```python
from build123d import *

# Parameters (mm, degrees)
EXTRUDE_1_DEPTH        = 8
SKETCH_2_W             = 101.5
SKETCH_2_H             = 90.5
PCB_DEPTH              = 1.62
CUT_EXTRUDE_1931_REACH = 77.575
SKETCH_2_4_W           = 102
SKETCH_2_4_H           = 61
SKETCH_2_5_W           = 107
SKETCH_2_5_H           = 68.5
CUT_EXTRUDE_1995_DEPTH = 5.85
SKETCH_3_W             = 101.5
SKETCH_3_H             = 14
CUT_EXTRUDE_2361_DEPTH = 2.5
SKETCH_3_3_W           = 46
SKETCH_3_3_H           = 2
CUT_EXTRUDE_2_DEPTH    = 2.5
SKETCH_2585_R          = 2.15
CUT_EXTRUDE_2883_DEPTH = 2.2
SKETCH_3_2_R           = 1.15
CUT_EXTRUDE_2937_DEPTH = 76.574880086
FILLET_1_R             = 3
SKETCH_2_6_R           = 0.625
LED_DEPTH              = 76.574880086
PCB_START              = -1.62
SKETCH_2_7_W           = 54
SKETCH_2_7_H           = 4
PCB_2_DEPTH            = 1.62


with BuildPart() as part:
    # 草图1 → 凸台-拉伸1 (new body)
    with BuildSketch(Plane(origin=(0, 0, 0), x_dir=(1, 0, 0), z_dir=(0, 1, 0))):
        Polygon((57, 45.25), (60, 45.25), (60, 42.25), (60, -42.25), (60, -45.25), (57, -45.25), (-57, -45.25), (-60, -45.25), (-60, -42.25), (-60, 42.25), (-60, 45.25), (-57, 45.25), align=None)
    extrude(amount=EXTRUDE_1_DEPTH)

    # 草图2 → PCB (cut)
    with BuildSketch(Plane(origin=(0, 8, 0), x_dir=(1, 0, 0), z_dir=(0, 1, 0))):
        with Locations((2.75, 0)):
            Rectangle(SKETCH_2_W, SKETCH_2_H)
    extrude(amount=-PCB_DEPTH, mode=Mode.SUBTRACT)

    # 草图2<4> → Cut-Extrude 1931 (cut, up to next)
    with BuildSketch(Plane(origin=(0, 8, 0), x_dir=(1, 0, 0), z_dir=(0, 1, 0)), mode=Mode.PRIVATE) as cut_extrude_1931_sk1:
        with Locations((0, -5.25)):
            Rectangle(SKETCH_2_4_W, SKETCH_2_4_H)
    cut_extrude_1931_tool1 = extrude(cut_extrude_1931_sk1.sketch, amount=-CUT_EXTRUDE_1931_REACH, mode=Mode.PRIVATE) & part.part
    add(cut_extrude_1931_tool1.solids().sort_by_distance((0, 8, 5.25))[0], mode=Mode.SUBTRACT)

    # 草图2<5> → Cut-Extrude 1995 (cut)
    with BuildSketch(Plane(origin=(0, 8, 0), x_dir=(1, 0, 0), z_dir=(0, 1, 0))):
        with Locations((0, -7)):
            Rectangle(SKETCH_2_5_W, SKETCH_2_5_H)
    extrude(amount=-CUT_EXTRUDE_1995_DEPTH, mode=Mode.SUBTRACT)

    # Sketch 3 → Cut-Extrude 2361 (cut)
    with BuildSketch(Plane(origin=(0, 6.38, 0), x_dir=(1, 0, 0), z_dir=(0, 1, 0))):
        with Locations((2.75, 34.25)):
            Rectangle(SKETCH_3_W, SKETCH_3_H)
    extrude(amount=-CUT_EXTRUDE_2361_DEPTH, mode=Mode.SUBTRACT)

    # 草图3<3> → 穿孔焊盘切除2 (cut)
    with BuildSketch(Plane(origin=(0, 6.38, 0), x_dir=(1, 0, 0), z_dir=(0, 1, 0))):
        with Locations((-17, 42.25)):
            Rectangle(SKETCH_3_3_W, SKETCH_3_3_H)
    extrude(amount=-CUT_EXTRUDE_2_DEPTH, mode=Mode.SUBTRACT)

    # Sketch 2585 → Cut-Extrude 2883 (cut)
    with BuildSketch(Plane(origin=(0, 0, 0), x_dir=(1, 0, 0), z_dir=(0, 1, 0))):
        with Locations(Location((-56.5, -41.75, 0), (0, 0, 270))):
            Circle(SKETCH_2585_R)
        with Locations(Location((-56.5, 41.75, 0), (0, 0, 270))):
            Circle(SKETCH_2585_R)
        with Locations(Location((56.5, 41.75, 0), (0, 0, 270))):
            Circle(SKETCH_2585_R)
        with Locations(Location((56.5, -41.75, 0), (0, 0, 270))):
            Circle(SKETCH_2585_R)
    extrude(amount=CUT_EXTRUDE_2883_DEPTH, mode=Mode.SUBTRACT)

    # Sketch 3 2 → Cut-Extrude 2937 (cut, through all)
    with BuildSketch(Plane(origin=(0, 0, 0), x_dir=(1, 0, 0), z_dir=(0, 1, 0))):
        with Locations(Location((-56.5, -41.75, 0), (0, 0, 270))):
            Circle(SKETCH_3_2_R)
        with Locations(Location((-56.5, 41.75, 0), (0, 0, 270))):
            Circle(SKETCH_3_2_R)
        with Locations(Location((56.5, 41.75, 0), (0, 0, 270))):
            Circle(SKETCH_3_2_R)
        with Locations(Location((56.5, -41.75, 0), (0, 0, 270))):
            Circle(SKETCH_3_2_R)
    extrude(amount=CUT_EXTRUDE_2937_DEPTH, mode=Mode.SUBTRACT)

    # 圆角1
    # the kernel refuses this fillet: 3 mm, written as the material it adds along each edge
    with BuildSketch(Plane(origin=(-51, 2.15, -25.25), x_dir=(1, 0, 0), z_dir=(0, -1, 0)), Plane(origin=(-51, 2.15, 35.75), x_dir=(0, 0, -1), z_dir=(0, -1, 0))) as fillet_1_piece_1:
        with BuildLine():
            CenterArc((FILLET_1_R, FILLET_1_R), FILLET_1_R, 180, 90)
            Line((0, FILLET_1_R), (0, 0))
            Line((0, 0), (FILLET_1_R, 0))
        make_face()
    extrude(amount=2.15)
    with BuildSketch(Plane(origin=(-53.5, 8, -27.25), x_dir=(1, 0, 0), z_dir=(0, -1, 0))) as fillet_1_piece_2:
        with BuildLine():
            CenterArc((FILLET_1_R, FILLET_1_R), FILLET_1_R, 180, 90)
            Line((0, FILLET_1_R), (0, 0))
            Line((0, 0), (FILLET_1_R, 0))
        make_face()
    extrude(amount=5.85)
    with BuildSketch(Plane(origin=(-53.5, 8, 41.25), x_dir=(1, 0, 0), z_dir=(0, -1, 0))) as fillet_1_piece_3:
        with BuildLine():
            CenterArc((FILLET_1_R, -FILLET_1_R), FILLET_1_R, 90, 90)
            Line((0, -FILLET_1_R), (0, 0))
            Line((0, 0), (FILLET_1_R, 0))
        make_face()
    extrude(amount=5.85)
    with BuildSketch(Plane(origin=(51, 2.15, 35.75), x_dir=(0, 0, -1), z_dir=(0, -1, 0)), Plane(origin=(51, 2.15, -25.25), x_dir=(-1, 0, 0), z_dir=(0, -1, 0))) as fillet_1_piece_4:
        with BuildLine():
            CenterArc((FILLET_1_R, -FILLET_1_R), FILLET_1_R, 90, 90)
            Line((0, -FILLET_1_R), (0, 0))
            Line((0, 0), (FILLET_1_R, 0))
        make_face()
    extrude(amount=2.15)
    with BuildSketch(Plane(origin=(53.5, 6.38, 41.25), x_dir=(0, 0, -1), z_dir=(0, -1, 0))) as fillet_1_piece_5:
        with BuildLine():
            CenterArc((FILLET_1_R, -FILLET_1_R), FILLET_1_R, 90, 90)
            Line((0, -FILLET_1_R), (0, 0))
            Line((0, 0), (FILLET_1_R, 0))
        make_face()
    extrude(amount=4.23)
    with BuildSketch(Plane(origin=(53.5, 3.88, -27.25), x_dir=(0, 0, 1), z_dir=(0, -1, 0))) as fillet_1_piece_6:
        with BuildLine():
            CenterArc((FILLET_1_R, FILLET_1_R), FILLET_1_R, 180, 90)
            Line((0, FILLET_1_R), (0, 0))
            Line((0, 0), (FILLET_1_R, 0))
        make_face()
    extrude(amount=1.73)
    with BuildSketch(Plane(origin=(6, 6.38, -43.25), x_dir=(-1, 0, 0), z_dir=(0, -1, 0))) as fillet_1_piece_7:
        with BuildLine():
            CenterArc((2.828427125, -3), FILLET_1_R, 90, 70.528779366)
            Line((0, -2), (0, 0))
            Line((0, 0), (2.828427125, 0))
        make_face()
    extrude(amount=2.5)
    with BuildSketch(Plane(origin=(-40, 6.38, -43.25), x_dir=(0, 0, 1), z_dir=(0, -1, 0))) as fillet_1_piece_8:
        with BuildLine():
            CenterArc((3, -2.828427125), FILLET_1_R, 109.471220634, 70.528779366)
            Line((0, -2.828427125), (0, 0))
            Line((0, 0), (2, 0))
        make_face()
    extrude(amount=2.5)
    with BuildSketch(Plane(origin=(-48, 6.38, -41.25), x_dir=(0, 0, 1), z_dir=(0, -1, 0))) as fillet_1_piece_9:
        with BuildLine():
            CenterArc((FILLET_1_R, -FILLET_1_R), FILLET_1_R, 90, 90)
            Line((0, -FILLET_1_R), (0, 0))
            Line((0, 0), (FILLET_1_R, 0))
        make_face()
    extrude(amount=2.5)
    with BuildSketch(Plane(origin=(53.5, 6.38, -41.25), x_dir=(0, 0, 1), z_dir=(0, -1, 0))) as fillet_1_piece_10:
        with BuildLine():
            CenterArc((FILLET_1_R, FILLET_1_R), FILLET_1_R, 180, 90)
            Line((0, FILLET_1_R), (0, 0))
            Line((0, 0), (FILLET_1_R, 0))
        make_face()
    extrude(amount=2.5)

    # 草图2<6> → LED孔 (cut, through all)
    with BuildSketch(Plane(origin=(0, 8, 0), x_dir=(1, 0, 0), z_dir=(0, 1, 0))):
        with Locations(Location((0.295, 40.636, 0), (0, 0, 270))):
            Circle(SKETCH_2_6_R)
        with Locations(Location((-27.9, 40.636, 0), (0, 0, 270))):
            Circle(SKETCH_2_6_R)
    extrude(amount=-LED_DEPTH, mode=Mode.SUBTRACT)

    # 草图2<7> → PCB 2 (add)
    with BuildSketch(Plane(origin=(0, 8, 0), x_dir=(1, 0, 0), z_dir=(0, 1, 0)).offset(PCB_START)):
        with Locations((8.5, -43.25)):
            Rectangle(SKETCH_2_7_W, SKETCH_2_7_H)
    extrude(amount=PCB_2_DEPTH)


solid = part.part
```
Work out the finished part from the listing and answer in its coordinate system (mm). A direction names the side the tool comes from. Round coordinates to 2 decimals unless told otherwise and drop trailing zeros. Loops run counter-clockwise (first coordinate to the right, second up) from the corner with the lowest first, then second, coordinate; pieces in that order, holes last.
(1) The part is cut by section D-D, the plane x = 43. Give the vertices of the cut face in (y, z), and give its area (3 significant figures).
Computed values:
outline: (0, -45.25) - (6.38, -45.25) - (6.38, -41.25) - (3.88, -41.25) - (3.88, -27.25) - (2.15, -27.25) - (2.15, -25.25) - (0, -25.25) - close; (0, 35.75) - (2.15, 35.75) - (2.15, 41.25) - (6.38, 41.25) - (6.38, 45.25) - (0, 45.25) - close
area: 121 mm2
(2) For faces 3 (the flat face through (-33, 6.38, 43)), 4 (the flat face through (53.5, 5, 1)), 5 (the cylindrical face through (-55.85, 1.08, 43.8)), 6 (the flat face through (1, 3, -45.25)), 7 (the cylindrical face through (50.1, 1.09, -24.39)), determine the directions among +Z, -Z, +X, -X, +Y, -Y from which every point of the face is accessible in a straight line to the end or side of a thin tool.
Computed values:
face 3: +Z, -Z, +Y
face 4: +Y
face 5: -Y
face 6: -Z, +X, -X, +Y, -Y
face 7: +Y, -Y
(3) The part is cut by section C-C, the plane z = -30.5. Give the vertices of the cut face in (x, y), and give its area (3 significant figures).
Computed values:
outline: (-60, 0) - (60, 0) - (60, 8) - (53.5, 8) - (53.5, 3.88) - (-48, 3.88) - (-48, 8) - (-60, 8) - close
area: 542 mm2
(4) Each of these flat-tipped pins is pushed along its axis until it touches: P1, Ø3, axis at x = -3, z = -27.5, coming from the +Y side; P2, Ø3, axis at x = -28, z = 42.5, coming from the +Y side; P3, Ø2.5, axis at x = -56.5, z = -41.75, coming from the -Y side; P4, Ø3.5, axis at x = -55.5, z = -42, coming from the -Y side. Where does it stop, or does it pass through?
Computed values:
P1: stops at y = 3.88
P2: stops at y = 6.38
P3: stops at y = 2.2
P4: stops at y = 0
(5) The mould has two halves that part along X. Classify faces 1 (the flat face through (56, 2.2, 43)), 2 (the flat face through (-1, 4, 45.25)): pulls with the +X half, pulls with the -X half, needs draft (parallel to the pull), parting line crosses it, or undercut.
Computed values:
face 1: undercut
face 2: needs draft
(6) Find the intervals of material crossed by L1, parallel to X at y = 3.55, z = -41.75; L2, parallel to X at y = 0.5, z = -41.75; L3, parallel to X at y = 5.25, z = 25, in increasing order.
Computed values:
L1: x = -60 to -57.65, -55.35 to 55.35, 57.65 to 60
L2: x = -60 to -58.65, -54.35 to 54.35, 58.65 to 60
L3: x = -60 to -53.5, 53.5 to 60
(7) The part is cut by section A-A, the plane x = -6. Give the vertices of the cut face in (y, z).
Computed values:
outline: (0, -45.25) - (6.38, -45.25) - (6.38, -43.25) - (3.88, -43.25) - (3.88, -27.25) - (2.15, -27.25) - (2.15, -25.25) - (0, -25.25) - close; (0, 35.75) - (2.15, 35.75) - (2.15, 41.25) - (8, 41.25) - (8, 45.25) - (0, 45.25) - close
(8) The part is cut by section B-B, the plane z = -8. Give the vertices of the cut face in (x, y), and give its area (3 significant figures).
Computed values:
outline: (-60, 0) - (-51, 0) - (-51, 2.15) - (-53.5, 2.15) - (-53.5, 8) - (-60, 8) - close; (51, 0) - (60, 0) - (60, 8) - (53.5, 8) - (53.5, 2.15) - (51, 2.15) - close
area: 115 mm2
